Part model, mm, in its own coordinate system. A direction names the side the tool comes from. Round coordinates to 2 decimals unless told otherwise and drop trailing zeros. Loops run counter-clockwise (first coordinate to the right, second up) from the corner with the lowest first, then second, coordinate; pieces in that order, holes last. Notation, with made-up numbers: M 53.5,-37 L 82.5,-37 A16 cw 82.5,-12 Z; hole C 23,-33.75 d7. An arc over 180 degrees is marked long. Answer as CSV lines item,"result". Start each with the question number.
Item 1: Band-saw the part on D-D (z = 2). Give the cut face in (x, y), and give its area (3 significant figures).
Item 2: Band-saw the part on B-B (x = 6). Give the cut face in (y, z).
Item 3: Wall check: line 1 (Y direction, x = 0, z = -2.25); line 2 (Y direction, x = 7, z = 1.25); line 3 (Y direction, x = 0.5, z = 3.25). Give the ranges that are in metal, low to high.
Item 4: Mould opens along Y. For faces 6 (the flat face through (-2.225, -3.178, 0.063)), 7 (the cylindrical face through (3.13, 4.4, 0.06)), 8 (the cylindrical face through (2.4, -0.07, 0.06)), 9 (the flat face through (3, -1, 5)) say: pulls with the +Y half, pulls with the -Y half, needs draft (parallel to the pull), parting line crosses it, or undercut.
Item 5: Band-saw the part on C-C (z = 4). Give the cut face in (x, y).
Item 6: Band-saw the part on A-A (y = 0). Give the cut face in (x, z), and give its area (3 significant figures).
Item 7: Drop flat-ended pins along their axis: pin 1 Ø3 at (x, y) = (6, 1) entering from -Z; pin 2 Ø1 at (x, z) = (-1.5, 2) entering from -Y; pin 3 Ø4 at (x, z) = (5, -0.5) entering from +Y; pin 4 Ø4 at (x, z) = (5.5, 0.5) entering from -Y. Give the stop position or say it passes through.
Item 8: Which spindle directions (+Z, -Z, +X, -X, +Y, -Y) get a long thin tool onto all of the face, cutting with end or side? Do faces 1 (the flat face through (-2.209, 3.155, 0.063)), 2 (the cylindrical face through (-2.11, 3.26, -4.85)), 3 (the flat face through (6, -3.5, 0)), 4 (the flat face through (6, 3.5, 0)), 5 (the cylindrical face through (-2.093, 3.238, 4.85)). Say none if no direction does.
```python
from build123d import *

# Parameters (mm, degrees)
EXTRUDE_THIN1_DEPTH = 5
FILLET1_R           = 0.6
FILLET2_R           = 0.5
BOSS_EXTRUDE1_START = 3.8
SKETCH2_W           = 5
SKETCH2_H           = 7
BOSS_EXTRUDE1_DEPTH = 4


with BuildPart() as part:
    # Sketch1 → Extrude-Thin1 (new, symmetric)
    with BuildSketch(Plane.XY):
        with BuildLine():
            ThreePointArc((-1.376583447, -1.965964906), (2.4, 0), (-1.376583447, 1.965964906))
            Line((-1.376583447, 1.965964906), (-3.097312756, 4.423421039))
            ThreePointArc((-3.097312756, 4.423421039), (5.4, 0), (-3.097312756, -4.423421039))
            Line((-3.097312756, -4.423421039), (-1.376583447, -1.965964906))
        make_face()
    extrude(amount=EXTRUDE_THIN1_DEPTH, both=True)

    # Fillet1
    fillet1_edges = [part.edges().sort_by_distance(p)[0] for p in [
        (2.4, 0, 5),
        (2.4, 0, -5),
        (5.4, 0, 5),
        (5.4, 0, -5),
    ]]
    fillet(fillet1_edges, radius=FILLET1_R)

    # Fillet2
    fillet2_edges = [part.edges().sort_by_distance(p)[0] for p in [
        (-2.236948102, -3.194692973, -5),
        (-2.236948102, 3.194692973, -5),
        (-1.376583447, 1.965964906, 0),
        (-2.236948102, 3.194692973, 5),
        (-3.097312756, 4.423421039, 0),
        (-2.996514767, 4.279466592, 4.824264069),
        (-2.996514767, 4.279466592, -4.824264069),
        (-1.477381436, 2.109919354, 4.824264069),
        (-1.477381436, 2.109919354, -4.824264069),
        (-1.376583447, -1.965964906, 0),
        (-3.097312756, -4.423421039, 0),
        (-2.236948102, -3.194692973, 5),
        (-2.996514767, -4.279466592, 4.824264069),
        (-2.996514767, -4.279466592, -4.824264069),
        (-1.477381436, -2.109919354, 4.824264069),
        (-1.477381436, -2.109919354, -4.824264069),
    ]]
    fillet(fillet2_edges, radius=FILLET2_R)

    # Sketch2 → Boss-Extrude1 (add)
    with BuildSketch(Plane(origin=(0, 0, 0), x_dir=(0, 0, -1), z_dir=(1, 0, 0)).offset(BOSS_EXTRUDE1_START)):
        Rectangle(SKETCH2_W, SKETCH2_H)
    extrude(amount=BOSS_EXTRUDE1_DEPTH)


solid = part.part
```
Answer block:
1,outline,"M -2.8,-3.99 A0.5 ccw -2.63,-4.72 A5.4 ccw 4.11,-3.5 L 7.8,-3.5 L 7.8,3.5 L 4.11,3.5 A5.4 ccw -2.63,4.72 A0.5 ccw -2.8,3.99 L -1.64,2.34 A0.5 ccw -1.02,2.17 A2.4 cw long -1.02,-2.17 A0.5 ccw -1.64,-2.34 Z"
1,area,"70.5 mm^2"
2,outline,"M -3.5,-2.5 L 3.5,-2.5 L 3.5,2.5 L -3.5,2.5 Z"
3,line 1,"y = -5.4 to -2.4, 2.4 to 5.4"
3,line 2,"y = -3.5 to 3.5"
3,line 3,"y = -5.38 to -2.35, 2.35 to 5.38"
4,face 6,"undercut"
4,face 7,"parting line crosses it"
4,face 8,"undercut"
4,face 9,"needs draft"
5,outline,"M -2.8,-3.99 A0.5 ccw -2.63,-4.72 A5.4 ccw long -2.63,4.72 A0.5 ccw -2.8,3.99 L -1.64,2.34 A0.5 ccw -1.02,2.17 A2.4 cw long -1.02,-2.17 A0.5 ccw -1.64,-2.34 Z"
6,outline,"M 2.4,-4.4 A0.6 ccw 3,-5 L 4.8,-5 A0.6 ccw 5.4,-4.4 L 5.4,-2.5 L 7.8,-2.5 L 7.8,2.5 L 5.4,2.5 L 5.4,4.4 A0.6 ccw 4.8,5 L 3,5 A0.6 ccw 2.4,4.4 Z"
6,area,"41.7 mm^2"
7,pin 1,"stops at z = -5"
7,pin 2,"stops at y = -5.31"
7,pin 3,"stops at y = 4.49"
7,pin 4,"stops at y = -4.11"
8,face 1,"+Z, -Z, -X"
8,face 2,"-Z, -X"
8,face 3,"+Z, -Z, +X, -Y"
8,face 4,"+Z, -Z, +X, +Y"
8,face 5,"+Z, -X"
